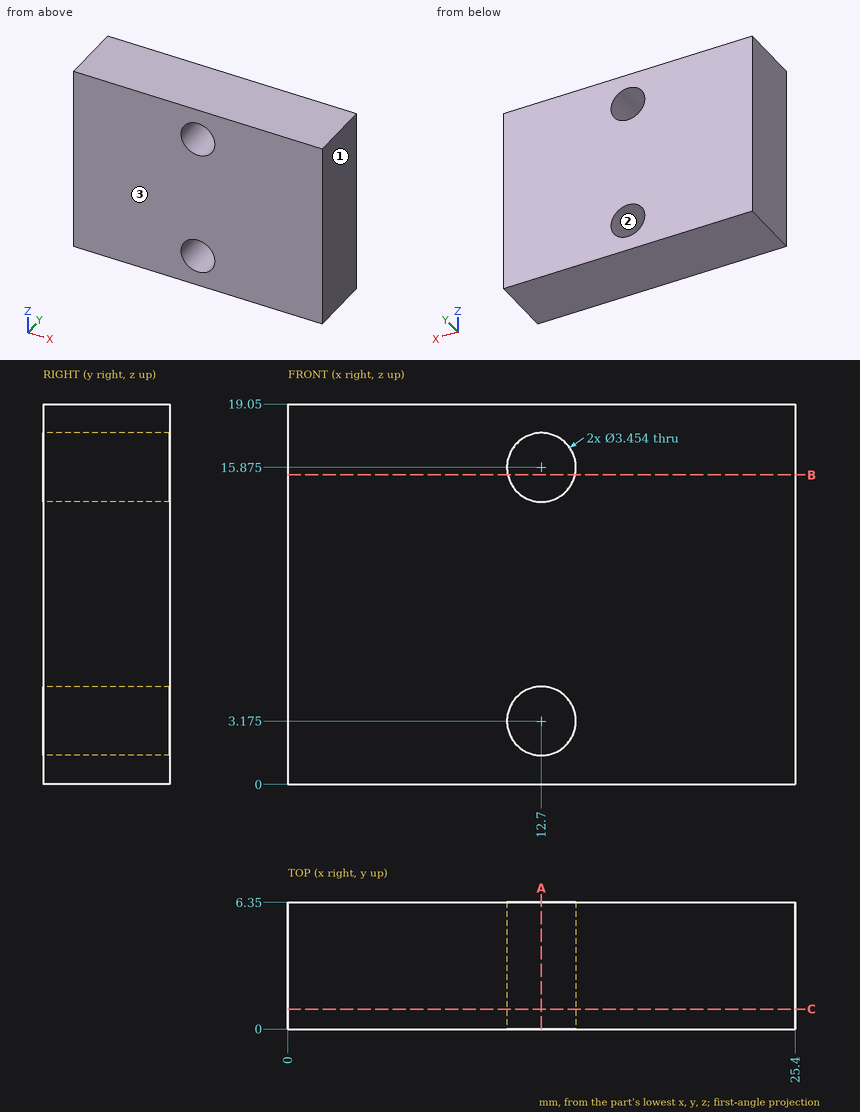
Geometry check sheet. Reference: drawing and pictorial views, mm from the part's lowest x, y, z. Give positions to 0.01 mm unless a question says otherwise; leave off trailing zeros. Order: outer loops, then holes, each group sorted by start corner. A loop starts at its lowest first (then second) coordinate and runs counter-clockwise, first axis right, second up. Notation, with made-up numbers: M 31.25,24.5 L 65.25,24.5 A9 ccw 65.25,32.5 Z; hole C -6,63.5 d11. An arc over 180 degrees is marked long. Use one line per item in the form item = value. Start each with the question number.
Q1. Scan lines: line 1 along Z through (x, y) = (12.7, 3); line 2 along X through (y, z) = (4.5, 16); line 3 along X through (y, z) = (5.75, 2.25). Record each from-to range of solid material in increasing order. Write a range as [from, to].
Q2. Section check A-A (x = 12.7). Enter the section's corners in (y, z).
Q3. Section check C-C (y = 1). Count the separate pieces of the cut face and the enclosed holes in it, then the cut area to 3 significant figures.
Q4. Section check B-B (z = 15.5). Enter the section's corners in (x, y), then the cut area to 3 significant figures.
Q5. Mould release check, pull along X, two halves, no side actions. Record for the marked faces 1, 2 and 3: +X half, -X half, draft (parallel to the pull), parting line (faces both ways), or undercut.
Q6. Go/stop test with a flat-tipped pin: pin 1 Ø3 at (x, z) = (12.7, 3.175) entering from -Y. Record where the tip stops, or that it passes through.
Evaluation:
q1.line_1 = [0, 1.45], [4.9, 14.15], [17.6, 19.05]
q1.line_2 = [0, 10.98], [14.42, 25.4]
q1.line_3 = [0, 11.24], [14.16, 25.4]
q2.outline = M 0,0 L 6.35,0 L 6.35,1.45 L 0,1.45 Z; M 0,4.9 L 6.35,4.9 L 6.35,14.15 L 0,14.15 Z; M 0,17.6 L 6.35,17.6 L 6.35,19.05 L 0,19.05 Z
q3.separate_pieces = 1
q3.enclosed_holes = 2
q3.area = 465 mm2
q4.outline = M 0,0 L 11.01,0 L 11.01,6.35 L 0,6.35 Z; M 14.39,0 L 25.4,0 L 25.4,6.35 L 14.39,6.35 Z
q4.area = 140 mm2
q5.face_1 = +X half
q5.face_2 = undercut
q5.face_3 = draft
q6.pin_1 = through
